Could you check a few things on this drawing? It's one solid part, dimensions in mm from its lowest x, y, z. A direction names the side the tool comes from. Give positions to 0.01 mm unless a question says otherwise; leave off trailing zeros. Order: outer loops, then holes, each group sorted by start corner. A loop starts at its lowest first (then second) coordinate and runs counter-clockwise, first axis right, second up.
Item 1: I'm going to push a flat-ended pin straight in: pin 1 Ø2 at (y, z) = (3, 27) entering from +X. Where does the tip first touch, or does it pass through?
Item 2: If I drill on line 1 along X through (y, z) = (2.5, 25.5); line 2 along X through (y, z) = (2, 5); line 3 along Y through (x, z) = (4.5, 3.5), over which ranges is the centre line in solid material (lowest first)?
Item 3: I want a section at B-B, the plane z = 19. Write out the boundary of the cut face in (x, y).
Item 4: I want a section at C-C, the plane x = 2.5. Write out the boundary of the cut face in (y, z), then the cut area to 3 significant figures.
Item 5: Which directions (+Z, -Z, +X, -X, +Y, -Y) give clear straight access to the entire face, cutting with the end or side of a thin tool? Please do the marked faces 5 and 6.
Item 6: If we mould it in two halves opening along Z, with no side actions, what happens to the marked faces 1, 2, 3 and 4? For each: +Z half, -Z half, draft (parallel to the pull), parting line (faces both ways), or undercut.
Item 7: I want a section at D-D, the plane z = 6. Write out the boundary of the cut face in (x, y) (1 decimal).
Item 8: I want a section at A-A, the plane y = 1.65. Write out the boundary of the cut face in (x, z).
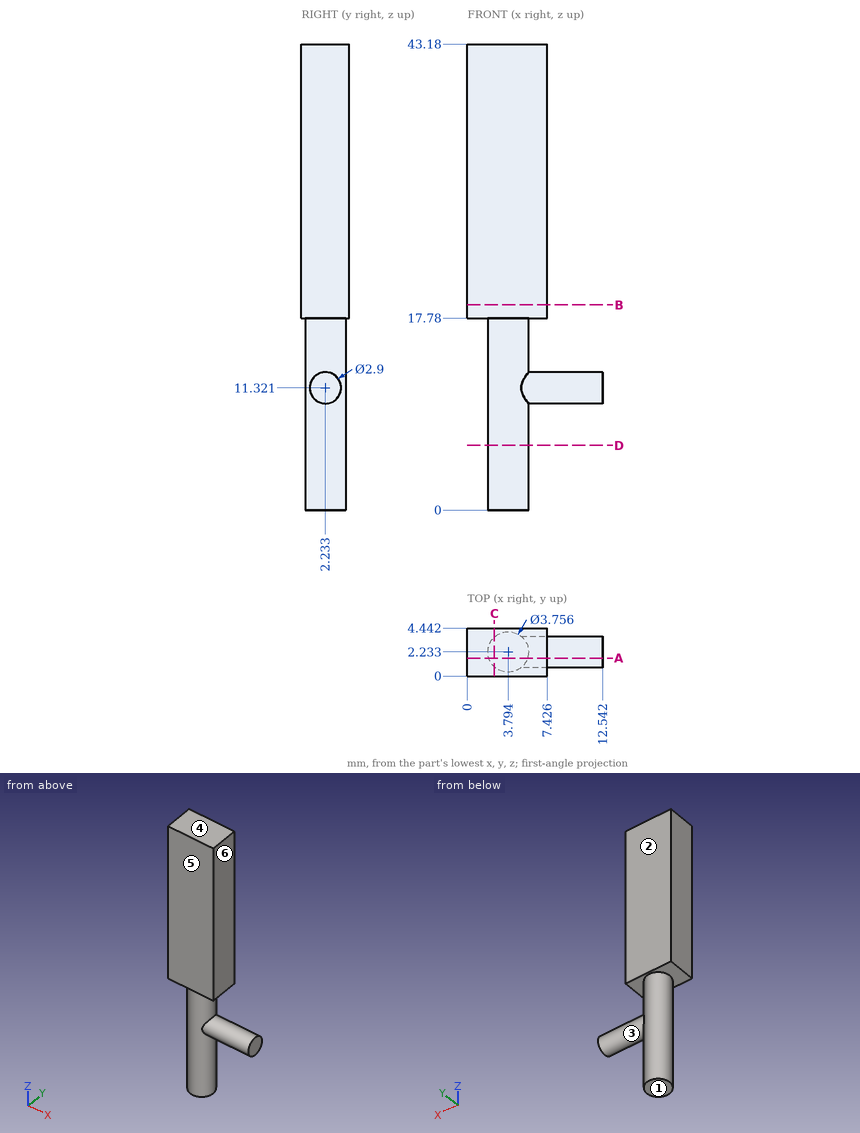
Results list:
1. pin 1: stops at x = 7.43
2. line 1: x = 0 to 7.43
2. line 2: x = 1.93 to 5.66
2. line 3: y = 0.49 to 3.97
3. outline: (0, 0) - (7.43, 0) - (7.43, 4.44) - (0, 4.44) - close
4. outline: (0, 17.78) - (0.87, 17.78) - (0.87, 0) - (3.59, 0) - (3.59, 17.78) - (4.44, 17.78) - (4.44, 43.18) - (0, 43.18) - close
4. area: 161 mm2
5. face 5: +Z, -Z, +X, -X, -Y
5. face 6: +Z, +X, +Y, -Y
6. face 1: -Z half
6. face 2: draft
6. face 3: undercut
6. face 4: +Z half
7. outline: circle Ø3.8 at (3.8, 2.2)
8. outline: (0, 17.78) - (2.01, 17.78) - (2.01, 0) - (5.58, 0) - (5.58, 9.99) - (12.54, 9.99) - (12.54, 12.65) - (5.58, 12.65) - (5.58, 17.78) - (7.43, 17.78) - (7.43, 43.18) - (0, 43.18) - close
